from build123d import *

# Parameters (mm, degrees)
SKETCH1_W           = 28.5
SKETCH1_H           = 21
BOSS_EXTRUDE1_DEPTH = 2
SKETCH2_W           = 1.5
SKETCH2_H           = 7
BOSS_EXTRUDE2_DEPTH = 6
SKETCH3_W           = 23.32
SKETCH3_H           = 7.76
BOSS_EXTRUDE3_DEPTH = 7.38
SKETCH4_R           = 2.472
CUT_EXTRUDE1_DEPTH  = 7.76
SKETCH5_R           = 3.1
CUT_EXTRUDE2_DEPTH  = 0.8
CUT_EXTRUDE3_START  = -0.8
SKETCH6_R           = 3.1
CUT_EXTRUDE3_DEPTH  = 0.8
FILLET1_R           = 3.69


with BuildPart() as part:
    # Sketch1 → Boss-Extrude1 (new body)
    with BuildSketch(Plane(origin=(0, 0, 0), x_dir=(1, 0, 0), z_dir=(0, 1, 0))):
        with Locations((14.25, 10.5)):
            Rectangle(SKETCH1_W, SKETCH1_H)
    extrude(amount=BOSS_EXTRUDE1_DEPTH)

    # Sketch2 → Boss-Extrude2 (add)
    with BuildSketch(Plane(origin=(0, 2, 0), x_dir=(1, 0, 0), z_dir=(0, 1, 0))):
        with Locations((2.75, 16)):
            Rectangle(SKETCH2_W, SKETCH2_H)
        with Locations((2.75, 5)):
            Rectangle(SKETCH2_W, SKETCH2_H)
        with Locations((25.75, 16)):
            Rectangle(SKETCH2_W, SKETCH2_H)
        with Locations((25.75, 5)):
            Rectangle(SKETCH2_W, SKETCH2_H)
    extrude(amount=BOSS_EXTRUDE2_DEPTH)

    # Sketch3 → Boss-Extrude3 (add)
    with BuildSketch(Plane.ZY):
        with Locations((-10.5, -1.88)):
            Rectangle(SKETCH3_W, SKETCH3_H)
    extrude(amount=BOSS_EXTRUDE3_DEPTH)

    # Sketch4 → Cut-Extrude1 (cut)
    with BuildSketch(Plane.XZ.offset(5.76)):
        with Locations(Location((-3.69, -2.53, 0), (0, 0, 270))):
            Circle(SKETCH4_R)
        with Locations(Location((-3.69, -10.5, 0), (0, 0, 270))):
            Circle(SKETCH4_R)
        with Locations(Location((-3.69, -18.47, 0), (0, 0, 270))):
            Circle(SKETCH4_R)
    extrude(amount=-CUT_EXTRUDE1_DEPTH, mode=Mode.SUBTRACT)

    # Sketch5 → Cut-Extrude2 (cut)
    with BuildSketch(Plane.XZ.offset(5.76)):
        with Locations(Location((-3.69, -2.53, 0), (0, 0, 270))):
            Circle(SKETCH5_R)
        with Locations(Location((-3.69, -10.5, 0), (0, 0, 270))):
            Circle(SKETCH5_R)
        with Locations(Location((-3.69, -18.47, 0), (0, 0, 270))):
            Circle(SKETCH5_R)
    extrude(amount=-CUT_EXTRUDE2_DEPTH, mode=Mode.SUBTRACT)

    # Sketch6 → Cut-Extrude3 (cut)
    with BuildSketch(Plane(origin=(0, 2, 0), x_dir=(1, 0, 0), z_dir=(0, 1, 0)).offset(CUT_EXTRUDE3_START)):
        with Locations(Location((-3.69, 10.5, 0), (0, 0, 90))):
            Circle(SKETCH6_R)
        with Locations(Location((-3.69, 18.47, 0), (0, 0, 90))):
            Circle(SKETCH6_R)
        with Locations(Location((-3.69, 2.53, 0), (0, 0, 90))):
            Circle(SKETCH6_R)
    extrude(amount=CUT_EXTRUDE3_DEPTH, mode=Mode.SUBTRACT)

    # Fillet1
    fillet1_edges = [part.edges().sort_by_distance(p)[0] for p in [
        (-7.38, -1.88, -22.16),
        (0, -1.88, -22.16),
        (0, -1.88, 1.16),
        (-7.38, -1.88, 1.16),
    ]]
    fillet(fillet1_edges, radius=FILLET1_R - 0.0001)  # a hair under: the kernel refuses the full size


solid = part.part
Here's how the part is built. I have some questions about the finished solid (model axes, mm). A direction names the side the tool comes from. Coordinates: 2 decimals unless noted, no trailing zeros. Write each loop counter-clockwise with the first axis right and the second up, starting at its lowest first coordinate (ties: lowest second). Pieces come first, ordered by that corner, then holes.
Item 1: On a 3-axis mill with a long thin cutter (end or side, diameter ignored), from which of +Z, -Z, +X, -X, +Y, -Y can I reach the whole of each face in a straight line? I mean faces 1 (the flat face through (25, 5, -16)), 2 (the flat face through (2, 5, -5)), 3 (the flat face through (3, 5, -8.5)), 4 (the flat face through (-5, -4.96, -8)), 5 (the flat face through (26, 5, -19.5)). Say none if no direction works.
Item 2: I want a section at A-A on z = -10.5. Write out the boundary of the cut face in (x, y), and give its area (3 significant figures).
Item 3: If I drill on line 1 (X direction, y = 1.55, z = -18.47); line 2 (X direction, y = 6, z = -7); line 3 (Y direction, x = -1, z = -16.5), over which ranges is the centre line in solid material (lowest first)?
Item 4: Will these pins go through, and if not, where does the flat tip stop? pin 1 (1.8 mm diameter, centred on y = 6.5, z = -4, fed in from -X); pin 2 (0.8 mm diameter, centred on x = 2.5, y = 5.5, fed in from +Z); pin 3 (8 mm diameter, centred on x = 15, z = -14.5, fed in from +Y); pin 4 (7 mm diameter, centred on x = -5, z = -2, fed in from -Y).
Item 5: I want a section at B-B on y = -3. Count the separate pieces of the cut face and the enclosed holes in it, and give its area (3 significant figures).
Item 6: I want a section at C-C on x = 5.5. Write out the boundary of the cut face in (y, z), and give its area (3 significant figures).
Item 7: If we mould it in two halves opening along Z, with no side actions, what happens to faces 6 (the flat face through (-2, -5.76, -13.3)), 7 (the cylindrical face through (-2.95, -1.92, -20.83)), 8 (the cylindrical face through (-6.27, -1.83, -21.11))? For each: +Z half, -Z half, draft (parallel to the pull), parting line (faces both ways), or undercut.
Item 8: I want a section at D-D on z = -3.75. Write out the boundary of the cut face in (x, y).
Findings below:
1. face 1: +Z, -Z, +Y
1. face 2: +Z, -Z, -X, +Y
1. face 3: +X, -X, +Y
1. face 4: -Y
1. face 5: -Z, +X, -X, +Y
2. outline: (-7.38, -5.76) - (-6.79, -5.76) - (-6.79, -4.96) - (-6.16, -4.96) - (-6.16, 1.2) - (-6.79, 1.2) - (-6.79, 2) - (-7.38, 2) - close; (-1.22, -4.96) - (-0.59, -4.96) - (-0.59, -5.76) - (0, -5.76) - (0, 0) - (28.5, 0) - (28.5, 2) - (-0.59, 2) - (-0.59, 1.2) - (-1.22, 1.2) - close
2. area: 73.9 mm2
3. line 1: x = -7.38 to -6.79, -0.59 to 28.5
3. line 2: x = 2 to 3.5, 25 to 26.5
3. line 3: y = -5.76 to 2
4. pin 1: stops at x = 2
4. pin 2: stops at z = -1.5
4. pin 3: stops at y = 2
4. pin 4: stops at y = -5.76
5. separate pieces: 1
5. enclosed holes: 3
5. area: 103 mm2
6. outline: (0, -21) - (2, -21) - (2, 0) - (0, 0) - close
6. area: 42.0 mm2
7. face 6: draft
7. face 7: undercut
7. face 8: -Z half
8. outline: (-7.38, -5.76) - (-6.54, -5.76) - (-6.54, -4.96) - (-5.84, -4.96) - (-5.84, 1.2) - (-6.54, 1.2) - (-6.54, 2) - (-7.38, 2) - close; (-1.54, -4.96) - (-0.84, -4.96) - (-0.84, -5.76) - (0, -5.76) - (0, 0) - (28.5, 0) - (28.5, 2) - (26.5, 2) - (26.5, 8) - (25, 8) - (25, 2) - (3.5, 2) - (3.5, 8) - (2, 8) - (2, 2) - (-0.84, 2) - (-0.84, 1.2) - (-1.54, 1.2) - close
